```python
from build123d import *

# Parameters (mm, degrees)
CROQUIS1_R              = 5.5
CROQUIS1_R_2            = 0.5
SALIENTE_EXTRUIR2_DEPTH = 3


with BuildPart() as part:
    # Croquis1 → Saliente-Extruir2 (new body)
    with BuildSketch(Plane(origin=(0, 0, 0), x_dir=(1, 0, 0), z_dir=(0, 1, 0))):
        with BuildLine():
            Line((-19.293466298, -8.829686884), (-17.293466298, -12.293788499))
            Line((-17.293466298, -12.293788499), (-5.259992013, -5.346258881))
            ThreePointArc((-5.259992013, -5.346258881), (0, -7.5), (5.259992013, -5.346258881))
            Line((5.259992013, -5.346258881), (17.293466298, -12.293788499))
            Line((17.293466298, -12.293788499), (19.293466298, -8.829686884))
            Line((19.293466298, -8.829686884), (7.259992013, -1.882157266))
            ThreePointArc((7.259992013, -1.882157266), (6.495190528, 3.75), (2, 7.228416147))
            Line((2, 7.228416147), (2, 21.123475383))
            Line((2, 21.123475383), (-2, 21.123475383))
            Line((-2, 21.123475383), (-2, 7.228416147))
            ThreePointArc((-2, 7.228416147), (-6.495190528, 3.75), (-7.259992013, -1.882157266))
            Line((-7.259992013, -1.882157266), (-19.293466298, -8.829686884))
        make_face()
        Circle(CROQUIS1_R, mode=Mode.SUBTRACT)
        with Locations((-13.423393759, -7.75)):
            Circle(CROQUIS1_R_2, mode=Mode.SUBTRACT)
        with Locations((0, 15.5)):
            Circle(CROQUIS1_R_2, mode=Mode.SUBTRACT)
        with Locations((13.423393759, -7.75)):
            Circle(CROQUIS1_R_2, mode=Mode.SUBTRACT)
    extrude(amount=SALIENTE_EXTRUIR2_DEPTH)


solid = part.part
```
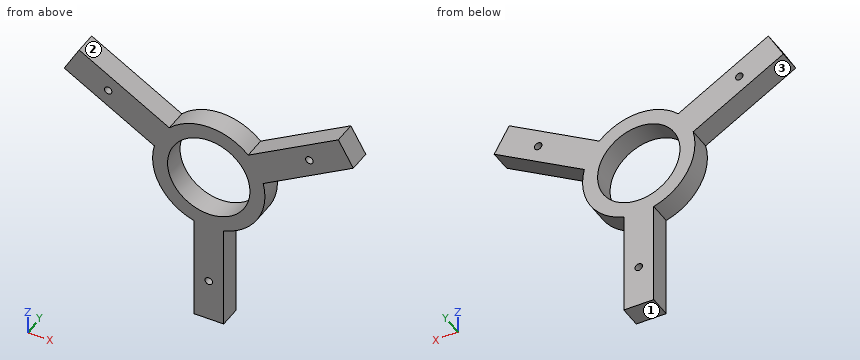
The listing builds one solid part. Answer for the finished solid, in the listing's coordinates (mm). Face numbers are marked on the shaded views. Give positions to 0.01 mm unless a question says otherwise; leave off trailing zeros. Order: outer loops, then holes, each group sorted by start corner. A loop starts at its lowest first (then second) coordinate and runs counter-clockwise, first axis right, second up.
1) Determine the mould class of the marked faces 1, 2 and 3 for opening direction X: pulls with the +X half, pulls with the -X half, needs draft (parallel to the pull), parting line crosses it, or undercut.
Reported:
face 1: needs draft
face 2: undercut
face 3: pulls with the -X half
2) Consider line 1 along X through (y, z) = (1.55, 0); line 2 along X through (y, z) = (1.45, 6); line 3 along X through (y, z) = (2.05, 7.75). Determine where each line is inside the solid, lowest interval first.
Reported:
line 1: x = -7.5 to -5.5, 5.5 to 7.5
line 2: x = -14.39 to -6.39, -4.5 to 4.5, 6.39 to 14.39
line 3: x = -17.42 to -13.92, -12.92 to -9.42, 9.42 to 12.92, 13.92 to 17.42
3) Find section B-B on x = 0. Write down the section's boundary in (y, z), then the cut area to 3 significant figures.
Reported:
outline: (0, -21.12) - (3, -21.12) - (3, -16) - (0, -16) - close; (0, -15) - (3, -15) - (3, -5.5) - (0, -5.5) - close; (0, 5.5) - (3, 5.5) - (3, 7.5) - (0, 7.5) - close
area: 49.9 mm2
4) Find section D-D on z = -15.5. Write down the section's boundary in (x, y), then the cut area to 3 significant figures.
Reported:
outline: (-2, 0) - (-0.5, 0) - (-0.5, 3) - (-2, 3) - close; (0.5, 0) - (2, 0) - (2, 3) - (0.5, 3) - close
area: 9.00 mm2
5) Find section A-A on z = 0. Write down the section's boundary in (x, y).
Reported:
outline: (-7.5, 0) - (-5.5, 0) - (-5.5, 3) - (-7.5, 3) - close; (5.5, 0) - (7.5, 0) - (7.5, 3) - (5.5, 3) - close
6) Given P1, Ø1, axis at x = -0.5, y = 1.5, coming from the +Z side; P2, Ø5, axis at x = 12, z = -1, coming from the +Y side; P3, Ø1, axis at x = 13.5, y = 2, coming from the -Z side; P4, Ø17.5, axis at x = 0, z = 0, coming from the +Y side, each flat-ended and moving along its own axis, determine where each tip first touches the part or whether it passes through.
Reported:
P1: stops at z = 7.5
P2: passes through
P3: stops at z = 5.2
P4: stops at y = 3
7) Find section C-C on y = 1.45. Write down the section's boundary in (x, z), then the cut area to 3 significant figures.
Reported:
outline: (-19.29, 8.83) - (-7.26, 1.88) arc R7.5 ccw to (-2, -7.23) - (-2, -21.12) - (2, -21.12) - (2, -7.23) arc R7.5 ccw to (7.26, 1.88) - (19.29, 8.83) - (17.29, 12.29) - (5.26, 5.35) arc R7.5 ccw to (-5.26, 5.35) - (-17.29, 12.29) - close; hole circle Ø1 at (-13.42, 7.75); hole circle Ø11 at (0, 0); hole circle Ø1 at (0, -15.5); hole circle Ø1 at (13.42, 7.75)
area: 244 mm2
